```python
from build123d import *

# Parameters (mm, degrees)
CROQUIS1_W              = 55
CROQUIS1_H              = 55
SALIENTE_EXTRUIR1_DEPTH = 5
CROQUIS2_W              = 30
CROQUIS2_H              = 2
CROQUIS2_W_2            = 2
CROQUIS2_H_2            = 30
SALIENTE_EXTRUIR2_DEPTH = 1.5
CROQUIS3_R              = 1.6
CORTAR_EXTRUIR1_DEPTH   = 5
CROQUIS6_W              = 10
CROQUIS6_H              = 10
CORTAR_EXTRUIR4_DEPTH   = 10
CROQUIS7_R              = 2.75
CORTAR_EXTRUIR5_DEPTH   = 3


with BuildPart() as part:
    # Croquis1 → Saliente-Extruir1 (new body)
    with BuildSketch(Plane(origin=(0, 0, 0), x_dir=(1, 0, 0), z_dir=(0, 1, 0))):
        with Locations((27.5, 27.5)):
            Rectangle(CROQUIS1_W, CROQUIS1_H)
    extrude(amount=SALIENTE_EXTRUIR1_DEPTH)

    # Croquis2 → Saliente-Extruir2 (add)
    with BuildSketch(Plane(origin=(0, 5, 0), x_dir=(1, 0, 0), z_dir=(0, 1, 0))):
        with Locations((27.5, 51.25)):
            Rectangle(CROQUIS2_W, CROQUIS2_H)
        with Locations((3.75, 27.5)):
            Rectangle(CROQUIS2_W_2, CROQUIS2_H_2)
        with Locations((51.25, 27.5)):
            Rectangle(CROQUIS2_W_2, CROQUIS2_H_2)
        with Locations((27.5, 3.75)):
            Rectangle(CROQUIS2_W, CROQUIS2_H)
    extrude(amount=SALIENTE_EXTRUIR2_DEPTH)

    # Croquis3 → Cortar-Extruir1 (cut)
    with BuildSketch(Plane(origin=(0, 5, 0), x_dir=(1, 0, 0), z_dir=(0, 1, 0))):
        with Locations(Location((9.5, 38.75, 0), (0, 0, 270))):
            Circle(CROQUIS3_R)
        with Locations(Location((9.5, 16.25, 0), (0, 0, 270))):
            Circle(CROQUIS3_R)
        with Locations(Location((45.5, 38.75, 0), (0, 0, 90))):
            Circle(CROQUIS3_R)
        with Locations(Location((45.5, 16.25, 0), (0, 0, 90))):
            Circle(CROQUIS3_R)
    extrude(amount=-CORTAR_EXTRUIR1_DEPTH, mode=Mode.SUBTRACT)

    # Croquis6 → Cortar-Extruir4 (cut)
    with BuildSketch(Plane(origin=(0, 5, 0), x_dir=(1, 0, 0), z_dir=(0, 1, 0))):
        with Locations((27.5, 27.5)):
            Rectangle(CROQUIS6_W, CROQUIS6_H)
    extrude(amount=-CORTAR_EXTRUIR4_DEPTH, mode=Mode.SUBTRACT)

    # Croquis7 → Cortar-Extruir5 (cut)
    with BuildSketch(Plane(origin=(0, 5, 0), x_dir=(1, 0, 0), z_dir=(0, 1, 0))):
        with Locations(Location((9.5, 38.75, 0), (0, 0, 270))):
            Circle(CROQUIS7_R)
        with Locations(Location((45.5, 38.75, 0), (0, 0, 270))):
            Circle(CROQUIS7_R)
        with Locations(Location((45.5, 16.25, 0), (0, 0, 270))):
            Circle(CROQUIS7_R)
        with Locations(Location((9.5, 16.25, 0), (0, 0, 270))):
            Circle(CROQUIS7_R)
    extrude(amount=-CORTAR_EXTRUIR5_DEPTH, mode=Mode.SUBTRACT)


solid = part.part
```
The model under review builds one solid part; all positions refer to its coordinate system, in mm. A direction names the side the tool comes from. Coordinates: 2 decimals unless noted, no trailing zeros. Write each loop counter-clockwise with the first axis right and the second up, starting at its lowest first coordinate (ties: lowest second). Pieces come first, ordered by that corner, then holes. Notation, with made-up numbers: (-32, 3) -> (-16, 3) arc R24 ccw to (-16, 27) -> close; hole circle Ø5 at (-34.75, 5.25). An arc over 180 degrees is marked (long way). One line per item, written item: value. Start each with the question number.
Q1. To check wall thickness, follow probe 1 along Z at (x, y) = (45.5, 1.3); probe 2 along X at (y, z) = (4.3, -38.75); probe 3 along X at (y, z) = (1, -16.25). State the ranges of each line that lie inside material, in increasing order.
Q2. Add section A-A, the plane y = 5.75. Give the boundary of the cut face in (x, z), then the cut area to 3 significant figures.
Q3. For faces 1 (the face through (22.5, 3, -27)), 2 (the face through (42.5, 6, -4)), 3 (the face through (47.359, 3.521, -40.777)), 4 (the face through (4, 6, -42.5)), 5 (the face through (4.75, 6, -27)), list the 3-axis set-ups (+Z, -Z, +X, -X, +Y, -Y) from which the entire face can be reached by the end or side of a thin tool; tool diameter is ignored.
Q4. Add section D-D, the plane x = 16. Give the boundary of the cut face in (y, z).
Q5. Clearance check with flat-ended pins moving along their axes: P1, Ø1.6, axis at y = 6, z = -30.5, coming from the +X side; P2, Ø3.5, axis at x = 9.5, z = -16.25, coming from the +Y side; P3, Ø12, axis at x = 17, z = -36, coming from the +Y side. State where each tip first meets the part, or that it passes through.
Q6. Add section C-C, the plane x = 45.5. Give the boundary of the cut face in (y, z), then the cut area to 3 significant figures.
Q7. Add section B-B, the plane z = -38.75. Give the boundary of the cut face in (x, y).
Q8. The part is to be moulded in two halves that separate along Z. For faces 6 (the face through (27, 6, -52.25)), 7 (the face through (21, 0, -28)), 8 (the face through (27, 3, -22.5)), say which applies: +Z half, -Z half, draft (parallel to the pull), parting line (faces both ways), or undercut.
Response:
1. probe 1: -55 to -40.35, -37.15 to -17.85, -14.65 to 0
1. probe 2: 0 to 6.75, 12.25 to 42.75, 48.25 to 55
1. probe 3: 0 to 7.9, 11.1 to 43.9, 47.1 to 55
2. outline: (2.75, -42.5) -> (4.75, -42.5) -> (4.75, -12.5) -> (2.75, -12.5) -> close; (12.5, -52.25) -> (42.5, -52.25) -> (42.5, -50.25) -> (12.5, -50.25) -> close; (12.5, -4.75) -> (42.5, -4.75) -> (42.5, -2.75) -> (12.5, -2.75) -> close; (50.25, -42.5) -> (52.25, -42.5) -> (52.25, -12.5) -> (50.25, -12.5) -> close
2. area: 240 mm²
3. face 1: +Y, -Y
3. face 2: +Z, -Z, +X, +Y
3. face 3: +Y
3. face 4: -Z, +X, -X, +Y
3. face 5: +Z, -Z, +Y
4. outline: (0, -55) -> (5, -55) -> (5, -52.25) -> (6.5, -52.25) -> (6.5, -50.25) -> (5, -50.25) -> (5, -4.75) -> (6.5, -4.75) -> (6.5, -2.75) -> (5, -2.75) -> (5, 0) -> (0, 0) -> close
5. P1: x = 52.25
5. P2: y = 2
5. P3: y = 5
6. outline: (0, -55) -> (5, -55) -> (5, -41.5) -> (2, -41.5) -> (2, -40.35) -> (0, -40.35) -> close; (0, -37.15) -> (2, -37.15) -> (2, -36) -> (5, -36) -> (5, -19) -> (2, -19) -> (2, -17.85) -> (0, -17.85) -> close; (0, -14.65) -> (2, -14.65) -> (2, -13.5) -> (5, -13.5) -> (5, 0) -> (0, 0) -> close
6. area: 229 mm²
7. outline: (0, 0) -> (7.9, 0) -> (7.9, 2) -> (6.75, 2) -> (6.75, 5) -> (4.75, 5) -> (4.75, 6.5) -> (2.75, 6.5) -> (2.75, 5) -> (0, 5) -> close; (11.1, 0) -> (43.9, 0) -> (43.9, 2) -> (42.75, 2) -> (42.75, 5) -> (12.25, 5) -> (12.25, 2) -> (11.1, 2) -> close; (47.1, 0) -> (55, 0) -> (55, 5) -> (52.25, 5) -> (52.25, 6.5) -> (50.25, 6.5) -> (50.25, 5) -> (48.25, 5) -> (48.25, 2) -> (47.1, 2) -> close
8. face 6: -Z half
8. face 7: draft
8. face 8: undercut
